```python
from build123d import *

# Parameters (mm, degrees)
SKETCH1_R           = 7
BOSS_EXTRUDE1_DEPTH = 11
SKETCH2_R           = 3
CUT_EXTRUDE1_DEPTH  = 11
SKETCH3_R           = 4
CUT_EXTRUDE2_DEPTH  = 11


with BuildPart() as part:
    # Sketch1 → Boss-Extrude1 (new body, symmetric)
    with BuildSketch(Plane(origin=(0, 0, 0), x_dir=(1, 0, 0), z_dir=(0, 1, 0))):
        Circle(SKETCH1_R)
    extrude(amount=BOSS_EXTRUDE1_DEPTH, both=True)

    # Sketch2 → Cut-Extrude1 (cut)
    with BuildSketch(Plane(origin=(0, 11, 0), x_dir=(1, 0, 0), z_dir=(0, 1, 0))):
        Circle(SKETCH2_R)
    extrude(amount=-CUT_EXTRUDE1_DEPTH, mode=Mode.SUBTRACT)

    # Sketch3 → Cut-Extrude2 (cut)
    with BuildSketch(Plane.XZ.offset(11)):
        Circle(SKETCH3_R)
    extrude(amount=-CUT_EXTRUDE2_DEPTH, mode=Mode.SUBTRACT)


solid = part.part
```
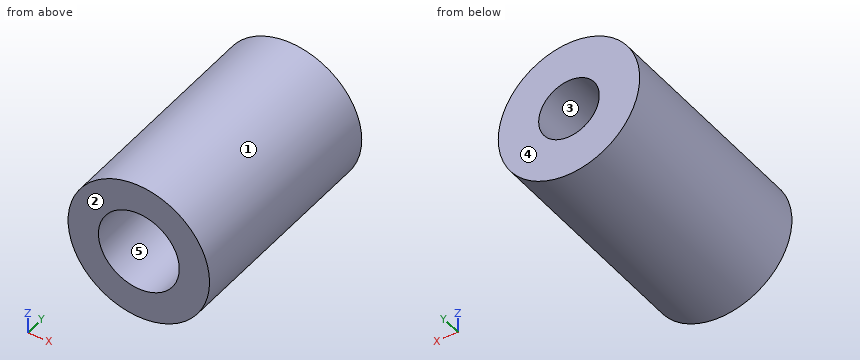
Could you check a few things on this model? Use its own coordinates, in mm. Face numbers are marked on the shaded views. A direction names the side the tool comes from. Give positions to 0.01 mm unless a question says otherwise; leave off trailing zeros. Write each loop counter-clockwise with the first axis right and the second up, starting at its lowest first coordinate (ties: lowest second). Pieces come first, ordered by that corner, then holes. Notation, with made-up numbers: (15, -15.5) - (26, -15.5) arc R37 cw to (26, 21.5) - close; hole circle Ø3 at (54.5, 58). An arc over 180 degrees is marked (long way). One line per item, written item: value. Start each with the question number.
Item 1: Imagine slicing it at C-C, the plane x = 3.25. List the corners of the cut face in (y, z) for me.
Item 2: Which directions (+Z, -Z, +X, -X, +Y, -Y) give clear straight access to the entire face, cutting with the end or side of a thin tool? Please do the marked faces 4 and 5.
Item 3: I'm going to push flat-ended pins straight in: pin 1 (6 mm diameter, centred on x = -3.5, y = -3.5, fed in from +Z); pin 2 (3 mm diameter, centred on x = 3.5, y = 0, fed in from -Z); pin 3 (2 mm diameter, centred on x = -4.5, y = 4.5, fed in from -Z). Where does each tip first touch, or does it pass through?
Item 4: Imagine slicing it at A-A, the plane x = 0. List the corners of the cut face in (y, z) for me.
Item 5: Please list where these lines run through material, in increasing order: line 1 (Z direction, x = 0, y = 7); line 2 (Z direction, x = 0, y = -7.75). Write a range as from..to.
Item 6: Imagine slicing it at D-D, the plane y = -3. List the corners of the cut face in (x, z) for me, and give its area (3 significant figures).
Item 7: Imagine slicing it at B-B, the plane z = 0. List the corners of the cut face in (x, y) for me, and give its area (3 significant figures).
Item 8: If we mould it in two halves opening along Z, with no side actions, what happens to the marked faces 1, 2 and 3? For each: +Z half, -Z half, draft (parallel to the pull), parting line (faces both ways), or undercut.
Geometry says:
1. outline: (-11, -6.2) - (11, -6.2) - (11, 6.2) - (-11, 6.2) - (-11, 2.33) - (0, 2.33) - (0, -2.33) - (-11, -2.33) - close
2. face 4: +Z, -Z, +X, -X, +Y
2. face 5: -Y
3. pin 1: z = 6.98
3. pin 2: z = -6.71
3. pin 3: z = -6.06
4. outline: (-11, -7) - (11, -7) - (11, -3) - (0, -3) - (0, -4) - (-11, -4) - close; (-11, 4) - (0, 4) - (0, 3) - (11, 3) - (11, 7) - (-11, 7) - close
5. line 1: -7..-3, 3..7
5. line 2: -7..-4, 4..7
6. outline: circle Ø14 at (0, 0); hole circle Ø8 at (0, 0)
6. area: 104 mm^2
7. outline: (-7, -11) - (-4, -11) - (-4, 0) - (-3, 0) - (-3, 11) - (-7, 11) - close; (3, 0) - (4, 0) - (4, -11) - (7, -11) - (7, 11) - (3, 11) - close
7. area: 154 mm^2
8. face 1: parting line
8. face 2: draft
8. face 3: undercut
